from build123d import *

# Parameters (mm, degrees)
SKETCH2_R           = 1.55
SKETCH2_R_2         = 2.499999997
SKETCH2_R_3         = 2.75
BOSS_EXTRUDE1_DEPTH = 5
CUT_EXTRUDE1_DEPTH  = 2


with BuildPart() as part:
    # Sketch2 → Boss-Extrude1 (new body)
    with BuildSketch(Plane.XY):
        with BuildLine():
            ThreePointArc((-12.525089607, -70.83564173), (-11.646409951, -72.956962073), (-9.525089607, -73.83564173))
            Line((-9.525089607, -73.83564173), (9.525089607, -73.83564173))
            ThreePointArc((9.525089607, -73.83564173), (11.646409951, -72.956962073), (12.525089607, -70.83564173))
            Line((12.525089607, -70.83564173), (12.525089607, -55.009940427))
            ThreePointArc((12.525089607, -55.009940427), (30.521330754, -47.449128385), (44.86389153, -34.208224921))
            add(Edge.make_bspline(
                [(78.006603773, -18.655919566), (58.043406574, -17.372955625), (44.86389153, -34.208224921)],
                knots=[0, 0, 0, 1, 1, 1], degree=2))
            Line((78.006603773, -18.655919566), (88.527931482, -18.655919566))
            ThreePointArc((88.527931482, -18.655919566), (98.717948133, -7.13841292), (88.716103535, 4.542875677))
            Line((88.716103535, 4.542875677), (69.795285346, 4.472063654))
            Line((69.795285346, 4.472063654), (44.465833223, 4.48880334))
            ThreePointArc((44.465833223, 4.48880334), (42.333815881, 3.601374029), (41.463969238, 1.462122864))
            Line((41.463969238, 1.462122864), (41.491086519, -1.586796959))
            ThreePointArc((41.491086519, -1.586796959), (42.375663318, -3.687434951), (44.481277596, -4.560100178))
            Line((44.481277596, -4.560100178), (47.998316287, -4.571460593))
            ThreePointArc((47.998316287, -4.571460593), (0, -48.215522587), (-47.998316287, -4.571460593))
            Line((-47.998316287, -4.571460593), (-44.481277596, -4.560100178))
            ThreePointArc((-44.481277596, -4.560100178), (-42.375663318, -3.687434951), (-41.491086519, -1.586796959))
            Line((-41.491086519, -1.586796959), (-41.463969238, 1.462122864))
            ThreePointArc((-41.463969238, 1.462122864), (-42.333815881, 3.601374029), (-44.465833223, 4.48880334))
            Line((-44.465833223, 4.48880334), (-48.006603773, 4.486463321))
            Line((-48.006603773, 4.486463321), (-77.006603773, 4.569081841))
            Line((-77.006603773, 4.569081841), (-87.006603773, 4.569081841))
            ThreePointArc((-87.006603773, 4.569081841), (-98.619104477, -7.043418862), (-87.006603773, -18.655919566))
            Line((-87.006603773, -18.655919566), (-78.006603773, -18.655919566))
            add(Edge.make_bspline(
                [(-78.006603773, -18.655919566), (-58.043406574, -17.372955625), (-44.86389153, -34.208224921)],
                knots=[0, 0, 0, 1, 1, 1], degree=2))
            ThreePointArc((-44.86389153, -34.208224921), (-30.521330754, -47.449128385), (-12.525089607, -55.009940427))
            Line((-12.525089607, -55.009940427), (-12.525089607, -70.83564173))
        make_face()
        with Locations((-87.006603773, -16.043418862)):
            Circle(SKETCH2_R, mode=Mode.SUBTRACT)
        with Locations((-96.006603773, -7.043418862)):
            Circle(SKETCH2_R, mode=Mode.SUBTRACT)
        with Locations((-87.006603773, -7.043418862)):
            Circle(SKETCH2_R_2, mode=Mode.SUBTRACT)
        with Locations((-78.006603773, -7.043418862)):
            Circle(SKETCH2_R, mode=Mode.SUBTRACT)
        with Locations((-87.006603773, 1.956581138)):
            Circle(SKETCH2_R, mode=Mode.SUBTRACT)
        with Locations((-46, 0)):
            Circle(SKETCH2_R, mode=Mode.SUBTRACT)
        with Locations((87.006603773, -16.043418862)):
            Circle(SKETCH2_R, mode=Mode.SUBTRACT)
        with Locations((46, 0)):
            Circle(SKETCH2_R, mode=Mode.SUBTRACT)
        with Locations((78.006603773, -7.043418862)):
            Circle(SKETCH2_R, mode=Mode.SUBTRACT)
        with Locations((87.006603773, -7.043418862)):
            Circle(SKETCH2_R_2, mode=Mode.SUBTRACT)
        with Locations((96.006603773, -7.043418862)):
            Circle(SKETCH2_R, mode=Mode.SUBTRACT)
        with Locations((87.006603773, 1.956581138)):
            Circle(SKETCH2_R, mode=Mode.SUBTRACT)
        with Locations((0, -61)):
            Circle(SKETCH2_R_3, mode=Mode.SUBTRACT)
    extrude(amount=BOSS_EXTRUDE1_DEPTH)

    # Sketch3 → Cut-Extrude1 (cut)
    with BuildSketch(Plane(origin=(0, 0, 0), x_dir=(-1, 0, 0), z_dir=(0, 0, -1))):
        with BuildLine():
            Line((9.5, -49.5), (-9.5, -49.5))
            ThreePointArc((-9.5, -49.5), (-10.914213562, -50.085786438), (-11.5, -51.5))
            Line((-11.5, -51.5), (-11.5, -70.5))
            ThreePointArc((-11.5, -70.5), (-10.914213562, -71.914213562), (-9.5, -72.5))
            Line((-9.5, -72.5), (9.5, -72.5))
            ThreePointArc((9.5, -72.5), (10.914213562, -71.914213562), (11.5, -70.5))
            Line((11.5, -70.5), (11.5, -51.5))
            ThreePointArc((11.5, -51.5), (10.914213562, -50.085786438), (9.5, -49.5))
        make_face()
    extrude(amount=-CUT_EXTRUDE1_DEPTH, mode=Mode.SUBTRACT)


solid = part.part
Geometry check sheet. Reference: the model listing, model coordinates, mm. A direction names the side the tool comes from. Round coordinates to 2 decimals unless told otherwise and drop trailing zeros. Loops run counter-clockwise (first coordinate to the right, second up) from the corner with the lowest first, then second, coordinate; pieces in that order, holes last. Notation, with made-up numbers: (69, -7) -> (97, -7) arc R15 ccw to (97, -1) -> close; hole circle Ø2 at (19.5, 7). An arc over 180 degrees is marked (long way). Answer as a JSON object with one key per item and string values. Group by question number.
Item 1: Cross-section at C-C, the plane y = -43. Record the cut outline in (x, z), plus the area to 3 significant figures.
Item 2: Release check for a two-part mould opening along Y. For faces 1 (the face through (89.316, -8.001, 2.465)), 2 (the face through (0, -73.836, 2)), 3 (the face through (-12.525, -63, 2)) record: pulls with the +Y half, pulls with the -Y half, needs draft (parallel to the pull), parting line crosses it, or undercut.
Item 3: Set-up check for faces 4 (the face through (-83, -18.656, 2)), 5 (the face through (83, -18.656, 2)), 6 (the face through (-98.616, -6.788, 2.465)), 7 (the face through (0.996, -48.205, 2.465)): record each of +Z, -Z, +X, -X, +Y, -Y from which the full face is reachable in a straight line by a thin tool's end or side.
Item 4: Thickness scan on line 1 along X through (y, z) = (-58, 1.6); line 2 along X through (y, z) = (-17, 4.65); line 3 along Y through (x, z) = (-86.5, 4.85). Record the ranges inside material, lowest first.
Item 5: Cross-section at D-D, the plane z = 4.05. Count the separate pieces of the cut face and the enclosed holes in it, plus the area to 3 significant figures.
Item 6: Cross-section at B-B, the plane x = 0. Record the cut outline in (y, z).
Item 7: Depth check by flat-ended pin: pin 1 Ø1 at (y, z) = (-42, 3) entering from -X; pin 2 Ø4 at (x, y) = (-26, -53.5) entering from -Z; pin 3 Ø4 at (x, y) = (78.01, -7.04) entering from -Z; pin 4 Ø3 at (x, z) = (1.5, 2.5) entering from +Y. Enter the tip coordinate at first touch or a pass-through.
Item 8: Cross-section at A-A, the plane y = -61. Record the cut outline in (x, z).
Determined:
{
 "1": {"outline": "(-36.52, 0) -> (-21.81, 0) -> (-21.81, 5) -> (-36.52, 5) -> close; (21.81, 0) -> (36.52, 0) -> (36.52, 5) -> (21.81, 5) -> close", "area": "147 mm²"},
 "2": {"face 1": "undercut", "face 2": "pulls with the -Y half", "face 3": "needs draft"},
 "3": {"face 4": "+Z, -Z, -X, -Y", "face 5": "+Z, -Z, +X, -Y", "face 6": "+Z, -Z, -X", "face 7": "+Z, -Z"},
 "4": {"line 1": "x = -12.53 to -11.5, 11.5 to 12.53", "line 2": "x = -92.98 to -88.23, -85.79 to -45.12, 45.12 to 85.79, 88.23 to 93.17", "line 3": "y = -18.66 to -17.51, -14.58 to -9.49, -4.6 to 0.49, 3.42 to 4.57"},
 "5": {"separate pieces": "1", "enclosed holes": "13", "area": "3,860 mm²"},
 "6": {"outline": "(-73.84, 0) -> (-72.5, 0) -> (-72.5, 2) -> (-63.75, 2) -> (-63.75, 5) -> (-73.84, 5) -> close; (-58.25, 2) -> (-49.5, 2) -> (-49.5, 0) -> (-48.22, 0) -> (-48.22, 5) -> (-58.25, 5) -> close"},
 "7": {"pin 1": "stops at x = -38.22", "pin 2": "passes through", "pin 3": "stops at z = 0", "pin 4": "stops at y = -48.12"},
 "8": {"outline": "(-12.53, 0) -> (-11.5, 0) -> (-11.5, 2) -> (-2.75, 2) -> (-2.75, 5) -> (-12.53, 5) -> close; (2.75, 2) -> (11.5, 2) -> (11.5, 0) -> (12.53, 0) -> (12.53, 5) -> (2.75, 5) -> close"}
}
